```python
from build123d import *

# Parameters (mm, degrees)
ESBO_O1_R                     = 40
ESBO_O1_R_2                   = 30
RESSALTO_EXTRUS_O1_DEPTH      = 50
ESBO_O2_R                     = 1.500000000000004
ESBO_O2_R_2                   = 1.4999999999999962
ESBO_O2_R_3                   = 1.5
ESBO_O2_R_4                   = 1.500000000000002
ESBO_O2_R_5                   = 1.5000000000000018
CORTE_EXTRUS_O1_DEPTH         = 10
CORTE_EXTRUS_O2_DEPTH         = 11.84997677
RESSALTO_EXTRUS_O2_DEPTH      = 26.849976769999998
RESSALTO_EXTRUS_O2_DEPTH_BACK = 10
REVOLU_O1_ANGLE               = 180.0000000000004
RESSALTO_EXTRUS_O5_DEPTH      = 5
RESSALTO_EXTRUS_O5_DEPTH_BACK = 2
ESBO_O10_R                    = 11
ESBO_O13_R                    = 8
CORTE_EXTRUS_O4_DEPTH         = 40
CORTE_EXTRUS_O5_DEPTH         = 120
FILETE1_R                     = 50
FILETE2_R                     = 50


# Read off the part's stored shape, not the designer's step: Limites1, Limites2, Limites-Corte1
with BuildPart() as part:
    # Esbo_o1 → Ressalto-extrus_o1 (new body)
    with BuildSketch(Plane(origin=(0, 0, 0), x_dir=(1, 0, 0), z_dir=(0, 1, 0))):
        with Locations(Location((0, 0, 0), (0, 0, 270))):
            Circle(ESBO_O1_R)
        with Locations(Location((0, 0, 0), (0, 0, 270))):
            Circle(ESBO_O1_R_2, mode=Mode.SUBTRACT)
    extrude(amount=RESSALTO_EXTRUS_O1_DEPTH)

    # Esbo_o2 → Corte-extrus_o1 (cut)
    with BuildSketch(Plane(origin=(0, 0, 0), x_dir=(-1, 0, 0), z_dir=(0, -1, 0))):
        with Locations(Location((-21.160269082529076, -29.124611797498083, 0), (0, 0, 90))):
            Circle(ESBO_O2_R)
        with Locations(Location((-34.23803458662555, -11.124611797498012, 0), (0, 0, 90))):
            Circle(ESBO_O2_R_2)
        with Locations(Location((-34.23803458662548, 11.124611797498257, 0), (0, 0, 90))):
            Circle(ESBO_O2_R_3)
        with Locations(Location((21.16026908252929, 29.124611797497916, 0), (0, 0, 90))):
            Circle(ESBO_O2_R_4)
        with Locations(Location((34.23803458662564, 11.124611797497778, 0), (0, 0, 90))):
            Circle(ESBO_O2_R_5)
        with Locations(Location((34.2380345866254, -11.124611797498495, 0), (0, 0, 90))):
            Circle(ESBO_O2_R_4)
    extrude(amount=-CORTE_EXTRUS_O1_DEPTH, mode=Mode.SUBTRACT)

    # Esbo_o3 → Corte-extrus_o2 (cut)
    with BuildSketch(Plane(origin=(0, 0, 0), x_dir=(-1, 0, 0), z_dir=(0, -1, 0))):
        with BuildLine():
            ThreePointArc((30.293924667807104, -13.087327008263706), (31.253408488730912, 10.59360457240701), (16.0923575286481, 28.810345870366824))
            Line((16.092357528648105, 28.810345870366824), (19.505887913512822, 34.921631358020406))
            ThreePointArc((19.505887913512836, 34.9216313580204), (8.030354378354186, 39.18562757642205), (-4.197370072970371, 39.77916646274194))
            Line((-4.19737007297038, 39.779166462741934), (-3.1480275547272187, 29.83437484705651))
            ThreePointArc((-3.148027554727219, 29.834374847056512), (29.911212101346653, 2.3063804170720696), (1.462902849126346, -29.964310692122016))
            Line((1.4629028491263463, -29.96431069212202), (1.9505371321681024, -39.952414256162704))
            ThreePointArc((1.9505371321681024, -39.952414256162704), (22.185986251539575, -33.283359416478625), (36.12685933386897, -17.171197822832383))
            Line((36.12685933386898, -17.171197822832383), (30.293924667807104, -13.087327008263708))
        make_face()
    extrude(amount=-CORTE_EXTRUS_O2_DEPTH, mode=Mode.SUBTRACT)

    # Esbo_o4 → Ressalto-extrus_o2 (add, two sides: drawn at the far end of the back side and taken through both)
    with BuildSketch(Plane(origin=(0, 11.84997677, 0), x_dir=(-1, 0, 0), z_dir=(0, -1, 0)).offset(-RESSALTO_EXTRUS_O2_DEPTH_BACK)):
        with BuildLine():
            Line((-4.008838628941714, -29.730947056007228), (-4.700362462642585, -27.60265553746198))
            ThreePointArc((-4.700362462642585, -27.60265553746198), (-8.119302431706847, 26.796957439651234), (19.23025849893697, -20.351834267801586))
            Line((19.23025849893697, -20.351834267801586), (19.909240802048483, -22.441526924121003))
            ThreePointArc((19.909240802048483, -22.441526924121003), (-8.745833795666464, 28.696870756557733), (-4.008838628941714, -29.730947056007228))
        make_face()
    extrude(amount=RESSALTO_EXTRUS_O2_DEPTH + RESSALTO_EXTRUS_O2_DEPTH_BACK)

    # Esbo_o9 → Revolu_o1 (revolve)
    with BuildSketch(Plane(origin=(0, 50, 0), x_dir=(1, 0, 0), z_dir=(0, 1, 0))):
        with BuildLine():
            Line((-40, 0), (-30, 0))
            ThreePointArc((-30, 0), (1.84e-15, 30), (30, 0))
            Line((30, 0), (40, 0))
            ThreePointArc((40, 0), (2.45e-15, 40), (-40, 0))
        make_face()
    revolve(axis=Axis((-40, 50, 0), (1, 0, 0)), revolution_arc=REVOLU_O1_ANGLE)

    # Esbo_o10 → Ressalto-extrus_o5 (add, two sides: drawn at the far end of the back side and taken through both)
    with BuildSketch(Plane(origin=(0, 90, 0), x_dir=(1, 0, 0), z_dir=(0, 1, 0)).offset(-RESSALTO_EXTRUS_O5_DEPTH_BACK)):
        with Locations(Location((0, 0, 0), (0, 0, 270))):
            Circle(ESBO_O10_R)
    extrude(amount=RESSALTO_EXTRUS_O5_DEPTH + RESSALTO_EXTRUS_O5_DEPTH_BACK)

    # Limites1 outline → Limites1 (revolve)
    with BuildSketch(Plane.XY):
        Polygon((11, 95), (10.5, 115), (0, 115), (0, 95), align=None)
    revolve(axis=Axis((0, 0, 0), (0, 1, 0)))

    # Esbo_o13 → Corte-extrus_o4 (cut)
    with BuildSketch(Plane(origin=(0, 115, 0), x_dir=(1, 0, 0), z_dir=(0, 1, 0))):
        with Locations(Location((0, 0, 0), (0, 0, 270))):
            Circle(ESBO_O13_R)
    extrude(amount=-CORTE_EXTRUS_O4_DEPTH, mode=Mode.SUBTRACT)

    # Esbo_o14 → Corte-extrus_o5 (cut)
    with BuildSketch(Plane(origin=(61.11285487653572, 0, -34.135303848647126), x_dir=(-0.487647197837817, 0, -0.8730407839505122), z_dir=(0.8730407839505123, 0, -0.48764719783781707))):
        Polygon((54.65634856725553, 88.45776904605881), (-53.65162953624658, 88.45776904605881), (-53.651629536246595, 28.457769046058818), (54.65634856725555, 28.457769046058818), align=None)
    extrude(amount=-CORTE_EXTRUS_O5_DEPTH, mode=Mode.SUBTRACT)


with BuildPart() as corte_extrus_o5_piece_1:
    # of the separate pieces the step leaves, piece 1, a body of its own (corte_extrus_o5_pieces)
    add(part.part.solids().sort_by_distance((0, 0, 40))[0])



with BuildPart() as corte_extrus_o5_piece_2:
    # of the separate pieces the step leaves, piece 2, a body of its own (corte_extrus_o5_pieces)
    add(part.part.solids().sort_by_distance((0, 88.457769046, 11))[0])


with BuildPart() as corte_extrus_o5_piece_1_1:
    add(corte_extrus_o5_piece_1.part)

    add(corte_extrus_o5_piece_2.part)  # Limites2 merges Corte-extrus_o5 piece 2
    # Limites2 outline → Limites2 (revolve)
    with BuildSketch(Plane.XY):
        Polygon((0, 88.457769046), (0, 28.457769046), (40, 28.457769046), (11, 88.457769046), align=None)
    revolve(axis=Axis((0, 0, 0), (0, 1, 0)))

    # Limites-Corte1 outline → Limites-Corte1 (revolve, cut)
    with BuildSketch(Plane.XY):
        Polygon((30, 28.457769046), (8, 88.457769046), (0, 88.457769046), (0, 28.457769046), align=None)
    revolve(axis=Axis((0, 0, 0), (0, 1, 0)), mode=Mode.SUBTRACT)

    # Filete1
    # the kernel refuses this fillet: 50 mm, written as the material it takes off along each edge
    with BuildSketch(Plane(origin=(0, 28.457769046058818, 0), x_dir=(-1.8e-16, 0, 1), z_dir=(1, 0, 1.8e-16))) as filete1_piece_1:
        with BuildLine():
            CenterArc((40 - FILETE1_R, FILETE1_R * 0.228994080214), FILETE1_R, 334.2039735055, 25.79602649449996)
            Line((40, FILETE1_R * 0.228994080214), (40, 0))
            Line((40, 0), (40 - FILETE1_R * 0.0996510471581, -FILETE1_R * 0.206174580326))
        make_face()
    revolve(axis=Axis((0, 28.457769046058818, 0), (0, -1, 0)), revolution_arc=270, mode=Mode.SUBTRACT)
    with BuildSketch(Plane(origin=(0, 28.457769046058818, 0), x_dir=(1, 0, 0), z_dir=(0, 0, -1))) as filete1_piece_2:
        with BuildLine():
            CenterArc((40 - FILETE1_R, FILETE1_R * 0.228994080214), FILETE1_R, 334.2039735055, 25.79602649449996)
            Line((40, FILETE1_R * 0.228994080214), (40, 0))
            Line((40, 0), (40 - FILETE1_R * 0.0996510471581, -FILETE1_R * 0.206174580326))
        make_face()
    revolve(axis=Axis((0, 28.457769046058818, 0), (0, -1, 0)), revolution_arc=90, mode=Mode.SUBTRACT)

    # Filete2
    # the kernel refuses this fillet: 50 mm, written as the material it adds along each edge
    with BuildSketch(Plane(origin=(0, 28.457769046058818, 0), x_dir=(-1.8e-16, 0, 1), z_dir=(1, 0, 1.8e-16))) as filete2_piece_1:
        with BuildLine():
            CenterArc((30 - FILETE2_R, FILETE2_R * 0.177553692487), FILETE2_R, 339.86369657175186, 20.136303428248137)
            Line((30.000000000000007, FILETE2_R * 0.177553692487), (30, 0))
            Line((30, 0), (30 - FILETE2_R * 0.0611236841134, -FILETE2_R * 0.166700956672))
        make_face()
    revolve(axis=Axis((0, 28.457769046058818, 0), (0, -1, 0)), revolution_arc=270)
    with BuildSketch(Plane(origin=(0, 28.457769046058818, 0), x_dir=(1, 0, 0), z_dir=(0, 0, -1))) as filete2_piece_2:
        with BuildLine():
            CenterArc((30 - FILETE2_R, FILETE2_R * 0.177553692487), FILETE2_R, 339.86369657175186, 20.136303428248137)
            Line((30.000000000000007, FILETE2_R * 0.177553692487), (30, 0))
            Line((30, 0), (30 - FILETE2_R * 0.0611236841134, -FILETE2_R * 0.166700956672))
        make_face()
    revolve(axis=Axis((0, 28.457769046058818, 0), (0, -1, 0)), revolution_arc=90)


solid = corte_extrus_o5_piece_1_1.part
```
Can you work these out from the model? Positions are in its coordinate system, mm. A direction names the side the tool comes from. Coordinates: 2 decimals unless noted, no trailing zeros. Loops run counter-clockwise (first coordinate to the right, second up) from the corner with the lowest first, then second, coordinate; pieces in that order, holes last. Notation, with made-up numbers: (61, 33) -> (104, 33) arc R18 ccw to (104, 50) -> close; hole circle Ø7 at (86.25, 7). An arc over 180 degrees is marked (long way). Put each result on its own line as item: value. Start each with the question number.
Q1. I want a section at C-C (y = 47). Write out the boundary of the cut face in (x, z).
Q2. I want a section at A-A (y = 8.5). Write out the boundary of the cut face in (x, z).
Q3. Thinking about a two-plate mould opening in Y: for faces 1 (the face through (13, 21.85, -25)), 2 (the face through (3.68, 5.84, -34.88)), 3 (the face through (30, 0, -3.03)), which applies, pulls with the +Y half, pulls with the -Y half, needs draft (parallel to the pull), parting line crosses it, or undercut?
Q4. I want a section at B-B (y = 85). Write out the boundary of the cut face in (x, z), plus the area to 3 significant figures.
Q5. For faces 4 (the face through (-1.703, 5.842, 34.888)), 5 (the face through (34, 10, 11)), 6 (the face through (-32, 0, -11)), which set-ups out of +Z, -Z, +X, -X, +Y, -Y let a thin tool reach every point of the face, with its end or its side?
Q6. I'm going to push flat-ended pins straight in: P1, Ø2.5, axis at x = 33.5, z = 12, coming from the -Y side; P2, Ø1.5, axis at x = -34.5, z = 11, coming from the -Y side; P3, Ø1.5, axis at y = 9.5, z = -12.5, coming from the +X side; P4, Ø1, axis at x = -9.5, z = -26, coming from the -Y side. Where does each tip first touch, or does it pass through?
Q7. If I drill on line 1 (X direction, y = 4, z = 13); line 2 (Z direction, x = -11, y = 67); line 3 (Z direction, x = -2, y = 54.5), over which ranges is the centre line in solid material (lowest first)? Write a range as [from, to].
Taken from the geometry:
1. outline: circle Ø62.08 at (0, 0); hole circle Ø46.4 at (0, 0)
2. outline: (-36.13, 17.17) arc R40 ccw to (-19.51, -34.92) -> (-16.09, -28.81) arc R33 cw to (-30.29, 13.09) -> close; (-19.91, 22.44) arc R30 ccw to (3.15, -29.83) -> (4.2, -39.78) arc R40 ccw to (-1.95, 39.95) -> (-1.46, 29.96) arc R30 cw to (4.01, 29.73) -> (4.7, 27.6) arc R28 cw (long way) to (-19.23, 20.35) -> close; hole circle Ø3 at (-34.24, -11.12); hole circle Ø3 at (-34.24, 11.12); hole circle Ø3 at (-21.16, -29.12); hole circle Ø3 at (21.16, 29.12); hole circle Ø3 at (34.24, -11.12); hole circle Ø3 at (34.24, 11.12)
3. face 1: undercut
3. face 2: needs draft
3. face 3: pulls with the -Y half
4. outline: circle Ø25.34 at (0, 0); hole circle Ø18.54 at (0, 0)
4. area: 235 mm2
5. face 4: -X, -Y
5. face 5: -Y
5. face 6: -Z, -X, -Y
6. P1: stops at y = 0
6. P2: stops at y = 10
6. P3: stops at x = 38.24
6. P4: stops at y = -15
7. line 1: x = [-37.83, -30.33], [-27.04, -24.8], [24.8, 37.83]
7. line 2: z = [-18.32, -11.44], [11.44, 18.32]
7. line 3: z = [-27.34, -20.35], [20.35, 27.34]
